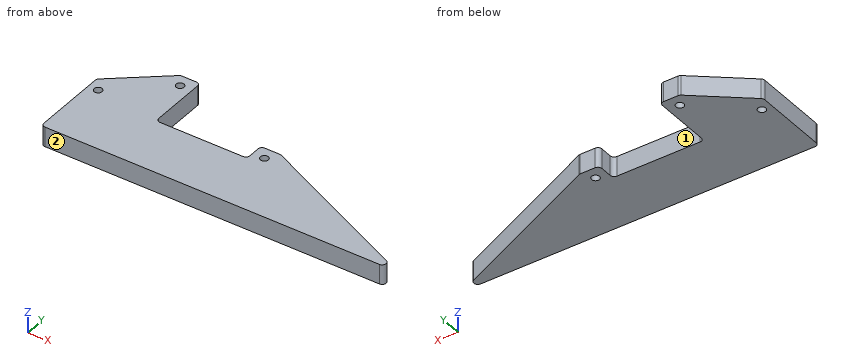
```python
from build123d import *

# Parameters (mm, degrees)
BOSS_EXTRUDE1_DEPTH      = 10
F_4_0_4_DIAMETER_HOLE1_D = 4
FILLET2_R                = 2


with BuildPart() as part:
    # Sketch1 → Boss-Extrude1 (new body)
    with BuildSketch(Plane.XY):
        Polygon((-87, 40), (0, 0), (-180, 0), (-180, 40), (-153, 62), (-143, 62), (-143, 30), (-97, 30), (-97, 40), align=None)
    extrude(amount=BOSS_EXTRUDE1_DEPTH)

    # Ø4.0 (4) Diameter Hole1 (through all)
    with Locations(Plane.XY.offset(10)):
        with Locations((-149, 56), (-91, 34), (-175, 34)):
            Hole(F_4_0_4_DIAMETER_HOLE1_D / 2)

    # Fillet2
    fillet2_edges = [part.edges().sort_by_distance(p)[0] for p in [
        (-153, 62, 5),
        (-143, 62, 5),
        (-143, 30, 5),
        (-97, 30, 5),
        (-97, 40, 5),
        (-87, 40, 5),
        (0, 0, 5),
        (-180, 0, 5),
        (-180, 40, 5),
    ]]
    fillet(fillet2_edges, radius=FILLET2_R)


solid = part.part
```
For this review, take the finished solid that the model builds, in its own axes (mm). Face numbers are marked on the shaded views. A direction names the side the tool comes from. Give positions to 0.01 mm unless a question says otherwise; leave off trailing zeros. Write each loop counter-clockwise with the first axis right and the second up, starting at its lowest first coordinate (ties: lowest second). Pieces come first, ordered by that corner, then holes. Notation, with made-up numbers: M -29.75,56.5 L 7.25,56.5 A22 cw 7.25,75.5 Z; hole C -34.75,69.5 d1. An arc over 180 degrees is marked long. Answer as a JSON object with one key per item and string values. Group by question number.
Item 1: For probe 1 along Y at (x, z) = (-91, 3); probe 2 along Y at (x, z) = (-118, 2.75); probe 3 along X at (y, z) = (57.5, 1), list the stretches that pass through material, from the lowest coordinate up. Write a range as [from, to].
Item 2: Consider section A-A on z = 4.75. Write out the cut boundary in (x, y), plus the area to 3 significant figures.
Item 3: Consider section D-D on y = 56. Write out the cut boundary in (x, z), plus the area to 3 significant figures.
Item 4: Consider section C-C on x = -91. Write out the cut boundary in (y, z), plus the area to 3 significant figures.
Item 5: For pin 1 Ø1.5 at (x, z) = (-110, 2) entering from +Y; pin 2 Ø3 at (y, z) = (38.5, 5) entering from +X (3 decimals); pin 3 Ø6 at (x, z) = (-90.5, 6.5) entering from +Y, all flat-tipped, find the tip position at first contact; note any pin that passes through.
Item 6: Tool access review of the marked faces 1 and 2: name each direction out of +Z, -Z, +X, -X, +Y, -Y from which nothing blocks a thin tool from reaching the whole face with its end or side.
Item 7: Consider section B-B on y = 34. Write out the cut boundary in (x, z), plus the area to 4 significant figures.
Check result:
{
 "1": {"probe 1": "y = [0, 32], [36, 40]", "probe 2": "y = [0, 30]", "probe 3": "x = [-158.52, -150.32], [-147.68, -143]"},
 "2": {"outline": "M -180,2 A2 ccw -178,0 L -9.14,0 A2 ccw -8.3,3.82 L -86.6,39.82 A2 ccw -87.44,40 L -95,40 A2 ccw -97,38 L -97,32 A2 cw -99,30 L -141,30 A2 cw -143,32 L -143,60 A2 ccw -145,62 L -152.29,62 A2 ccw -153.55,61.55 L -179.26,40.6 A2 ccw -180,39.05 Z; hole C -175,34 d4; hole C -149,56 d4; hole C -91,34 d4", "area": "5,470 mm^2"},
 "3": {"outline": "M -160.36,0 L -151,0 L -151,10 L -160.36,10 Z; M -147,0 L -143,0 L -143,10 L -147,10 Z", "area": "134 mm^2"},
 "4": {"outline": "M 0,0 L 32,0 L 32,10 L 0,10 Z; M 36,0 L 40,0 L 40,10 L 36,10 Z", "area": "360 mm^2"},
 "5": {"pin 1": "stops at y = 30", "pin 2": "stops at x = -80.475", "pin 3": "stops at y = 40"},
 "6": {"face 1": "+Z, -Z, +Y", "face 2": "+Z, -Z, +X, -X, -Y"},
 "7": {"outline": "M -180,0 L -177,0 L -177,10 L -180,10 Z; M -173,0 L -143,0 L -143,10 L -173,10 Z; M -97,0 L -93,0 L -93,10 L -97,10 Z; M -89,0 L -73.95,0 L -73.95,10 L -89,10 Z", "area": "520.5 mm^2"}
}
